Read the model definition and answer for the solid it produces. Units are mm, in the model's axes. A direction names the side the tool comes from. Coordinates: 2 decimals unless noted, no trailing zeros. Loops run counter-clockwise (first coordinate to the right, second up) from the corner with the lowest first, then second, coordinate; pieces in that order, holes last.
from build123d import *

# Parameters (mm, degrees)
SKETCH_1_W          = 97.6
SKETCH_1_H          = 97.6
SKETCH_1_R          = 1.59
EXTRUDE_1_DEPTH     = 2
SKETCH_2_R          = 1
CUT_EXTRUDE_1_DEPTH = 139.04173282
SKETCH_7_W          = 2.5
SKETCH_7_H          = 23.8
EXTRUDE_2_DEPTH     = 25
SKETCH_8_R          = 1.5
CUT_EXTRUDE_2_DEPTH = 141.643236595


with BuildPart() as part:
    # Эскиз1 → Бобышка-Вытянуть1 (new body)
    with BuildSketch(Plane(origin=(0, 0, 0), x_dir=(1, 0, 0), z_dir=(0, 1, 0))):
        with Locations((48.8, 48.8)):
            Rectangle(SKETCH_1_W, SKETCH_1_H)
        with Locations(Location((86.265001451, 91.665000306, 0), (0, 0, 270))):
            Circle(SKETCH_1_R, mode=Mode.SUBTRACT)
        with Locations(Location((88.805001451, 5.935000306, 0), (0, 0, 270))):
            Circle(SKETCH_1_R, mode=Mode.SUBTRACT)
        with Locations(Location((8.795001451, 5.935000306, 0), (0, 0, 270))):
            Circle(SKETCH_1_R, mode=Mode.SUBTRACT)
        with Locations(Location((12.605001451, 91.665000306, 0), (0, 0, 270))):
            Circle(SKETCH_1_R, mode=Mode.SUBTRACT)
        with BuildLine():
            Line((79.576520776, 92.6), (19.293482126, 92.6))
            ThreePointArc((19.293482126, 92.6), (17.512330868, 92.014021582), (16.426990408, 90.485000131))
            ThreePointArc((16.426990408, 90.485000131), (13.697675352, 87.817135476), (9.97357205, 88.652430089))
            ThreePointArc((9.97357205, 88.652430089), (6.759176917, 89.124368033), (5, 86.393002427))
            Line((5, 86.393002427), (5, 12.889708976))
            ThreePointArc((5, 12.889708976), (6.002770009, 10.651166513), (8.340714907, 9.909119546))
            ThreePointArc((8.340714907, 9.909119546), (10.982952752, 9.28356255), (12.616990516, 7.115000131))
            ThreePointArc((12.616990516, 7.115000131), (13.702330946, 5.5859785), (15.483482314, 5))
            Line((15.483482314, 5), (82.116520587, 5))
            ThreePointArc((82.116520587, 5), (83.897671955, 5.5859785), (84.983012386, 7.115000131))
            ThreePointArc((84.983012386, 7.115000131), (86.617049451, 9.283562094), (89.259286336, 9.909119736))
            ThreePointArc((89.259286336, 9.909119736), (91.597230458, 10.651167261), (92.6, 12.889709308))
            Line((92.6, 12.889709308), (92.6, 85.510507258))
            ThreePointArc((92.6, 85.510507258), (91.13495028, 88.088089), (88.170714907, 88.148147136))
            ThreePointArc((88.170714907, 88.148147136), (84.753959284, 87.961386993), (82.443012494, 90.485000131))
            ThreePointArc((82.443012494, 90.485000131), (81.357672034, 92.014021582), (79.576520776, 92.6))
        make_face(mode=Mode.SUBTRACT)
    extrude(amount=EXTRUDE_1_DEPTH)

    # Эскиз2 → Вырез-Вытянуть1 (cut, through all)
    with BuildSketch(Plane(origin=(0, 2, 0), x_dir=(1, 0, 0), z_dir=(0, 1, 0))):
        with Locations(Location((46.8, 95.1, 0), (0, 0, 270))):
            Circle(SKETCH_2_R)
        with Locations(Location((50.8, 95.1, 0), (0, 0, 90))):
            Circle(SKETCH_2_R)
    extrude(amount=-CUT_EXTRUDE_1_DEPTH, mode=Mode.SUBTRACT)

    # Эскиз7 → Бобышка-Вытянуть2 (add)
    with BuildSketch(Plane(origin=(0, 2, 0), x_dir=(1, 0, 0), z_dir=(0, 1, 0))):
        with Locations((1.25, 11.9)):
            Rectangle(SKETCH_7_W, SKETCH_7_H)
        with Locations((1.25, 85.7)):
            Rectangle(SKETCH_7_W, SKETCH_7_H)
        with Locations((96.35, 85.7)):
            Rectangle(SKETCH_7_W, SKETCH_7_H)
        with Locations((96.35, 11.9)):
            Rectangle(SKETCH_7_W, SKETCH_7_H)
    extrude(amount=EXTRUDE_2_DEPTH)

    # Эскиз8 → Вырез-Вытянуть2 (cut, through all)
    with BuildSketch(Plane.ZY):
        with Locations((-80.630070031, 19.32657333)):
            Circle(SKETCH_8_R)
        with Locations(Location((-90.769929969, 9.67342667, 0), (0, 0, 180))):
            Circle(SKETCH_8_R)
        with Locations((-6.830070031, 9.67342667)):
            Circle(SKETCH_8_R)
        with Locations(Location((-16.969929969, 19.32657333, 0), (0, 0, 180))):
            Circle(SKETCH_8_R)
    extrude(amount=-CUT_EXTRUDE_2_DEPTH, mode=Mode.SUBTRACT)


solid = part.part
Q1. Straight lines are drawn through the part: probe 1 along Z at (x, y) = (50.8, 0.65); probe 2 along X at (y, z) = (3, -78); probe 3 along X at (y, z) = (0.55, -95.1). For each, find the intervals that lie inside material, in ascending order.
Findings below:
probe 1: z = -97.6 to -96.1, -94.1 to -92.6, -5 to 0
probe 2: x = 0 to 2.5, 95.1 to 97.6
probe 3: x = 0 to 45.8, 47.8 to 49.8, 51.8 to 97.6
Q2. A cutting plane is placed at A-A (x = 76). Give the vertices of the cut face in (y, z), then the cut area to 3 significant figures.
Findings below:
outline: (0, -97.6) - (2, -97.6) - (2, -92.6) - (0, -92.6) - close; (0, -5) - (2, -5) - (2, 0) - (0, 0) - close
area: 20.0 mm2
Q3. A cutting plane is placed at B-B (z = -76). Give the vertices of the cut face in (x, y).
Findings below:
outline: (0, 0) - (5, 0) - (5, 2) - (2.5, 2) - (2.5, 27) - (0, 27) - close; (92.6, 0) - (97.6, 0) - (97.6, 27) - (95.1, 27) - (95.1, 2) - (92.6, 2) - close
Q4. Which of the six approach directions +Z, -Z, +X, -X, +Y, -Y give full straight-line access (tool end or side, diameter ignored) to faces 1 (the face through (96, 14, -23.8)), 2 (the face through (95.1, 14, -12)), 3 (the face through (17.534, 0.986, -92.03))?
Findings below:
face 1: +X, -X, +Y
face 2: +Z, -Z, +Y
face 3: +Y, -Y
Q5. Determine the mould class of faces 4 (the face through (96, 14, -73.8)), 5 (the face through (1.23, 19.39, -82.13)), 6 (the face through (96, 27, -86)) for opening direction Y: +Y half, -Y half, draft (parallel to the pull), parting line (faces both ways), or undercut.
Findings below:
face 4: draft
face 5: undercut
face 6: +Y half
Q6. A flat-ended cylindrical pin translates along its axis: pin 1 Ø1.5 at (y, z) = (4, -38) entering from +X. Find the tip coordinate at first contact, or state that the pin passes through.
Findings below:
pin 1: passes through
Q7. A cutting plane is placed at D-D (z = -61). Give the vertices of the cut face in (x, y).
Findings below:
outline: (0, 0) - (5, 0) - (5, 2) - (0, 2) - close; (92.6, 0) - (97.6, 0) - (97.6, 2) - (92.6, 2) - close
Q8. A cutting plane is placed at C-C (y = 13.5). Give the vertices of the cut face in (x, z), then the cut area to 3 significant figures.
Findings below:
outline: (0, -97.6) - (2.5, -97.6) - (2.5, -73.8) - (0, -73.8) - close; (0, -23.8) - (2.5, -23.8) - (2.5, 0) - (0, 0) - close; (95.1, -97.6) - (97.6, -97.6) - (97.6, -73.8) - (95.1, -73.8) - close; (95.1, -23.8) - (97.6, -23.8) - (97.6, 0) - (95.1, 0) - close
area: 238 mm2
